Verification items for this drawing (mm, ordinates from the low corner). A direction names the side the tool comes from. Round coordinates to 2 decimals unless told otherwise and drop trailing zeros. Order: outer loops, then holes, each group sorted by start corner. A loop starts at its lowest first (then second) coordinate and runs counter-clockwise, first axis right, second up. Notation, with made-up numbers: (5, 35) - (44, 35) arc R12 cw to (44, 47) - close; hole circle Ø5 at (84, 85). An arc over 180 degrees is marked (long way). One line per question, with ' | ' between items. Start each with the question number.
Q1. Gauge pin test, flat ends, axial feed: P1, Ø3, axis at x = 8, z = 5, coming from the -Y side; P2, Ø2.5, axis at x = 5.5, y = 2.5, coming from the +Z side. Record the tip position at first contact, or that the pin passes through.
Q2. Sectioned sample at C-C, the plane x = 12.25. Enter the section's corners in (y, z), then the cut area to 4 significant figures.
Q3. Sectioned sample at D-D, the plane z = 6.25. Enter the section's corners in (x, y), then the cut area to 3 significant figures.
Q4. Material ranges on line 1 along X through (y, z) = (1.65, 6.5); line 2 along Z through (x, y) = (15, 1.6), recorded low to high.
Q5. Sectioned sample at B-B, the plane y = 3.85. Enter the section's corners in (x, z).
Q6. Tool access check on the marked faces 1 and 2. Record the directions out of +Z, -Z, +X, -X, +Y, -Y that give a thin tool (end or side, any length) a straight path to the whole face; none if there is none.
Q7. Sectioned sample at A-A, the plane y = 0.45. Enter the section's corners in (x, z), then the cut area to 3 significant figures.
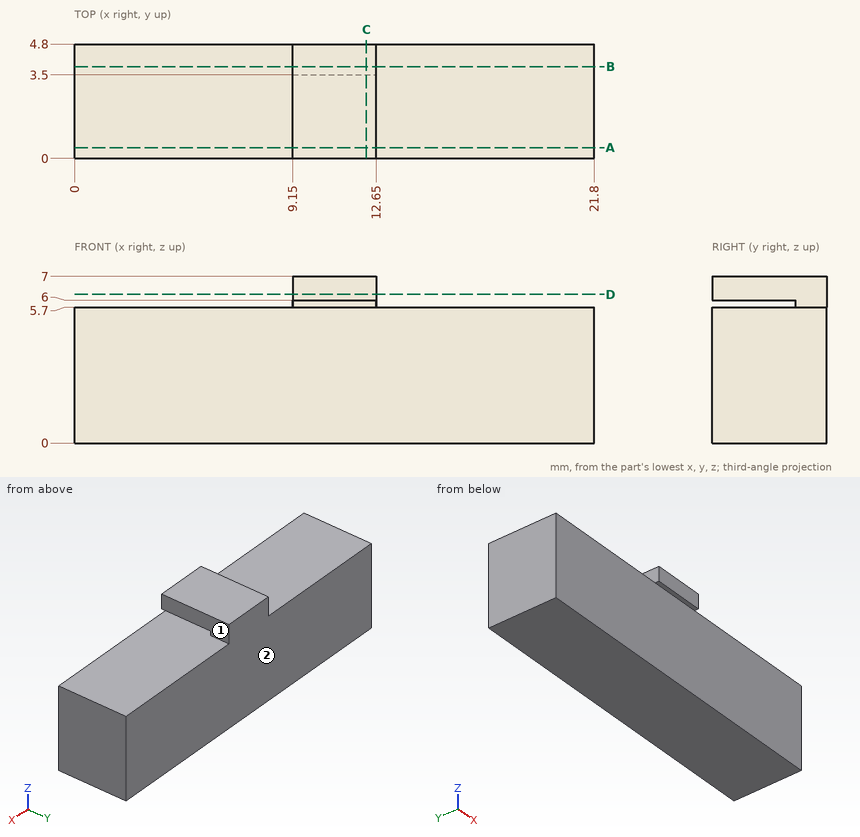
Determined:
1) P1: stops at y = 0 | P2: stops at z = 5.7
2) outline: (0, 0) - (4.8, 0) - (4.8, 7) - (0, 7) - (0, 6) - (3.5, 6) - (3.5, 5.7) - (0, 5.7) - close | area: 32.55 mm2
3) outline: (9.15, 0) - (12.65, 0) - (12.65, 4.8) - (9.15, 4.8) - close | area: 16.8 mm2
4) line 1: x = 9.15 to 12.65 | line 2: z = 0 to 5.7
5) outline: (0, 0) - (21.8, 0) - (21.8, 5.7) - (12.65, 5.7) - (12.65, 7) - (9.15, 7) - (9.15, 5.7) - (0, 5.7) - close
6) face 1: +Z, +X, +Y, -Y | face 2: +Z, -Z, +X, -X, +Y
7) outline: (0, 0) - (21.8, 0) - (21.8, 5.7) - (0, 5.7) - close; (9.15, 6) - (12.65, 6) - (12.65, 7) - (9.15, 7) - close | area: 128 mm2
